Can you work these out from the model? Positions are in its coordinate system, mm. Face numbers are marked on the shaded views. Give positions to 0.01 mm unless a question says otherwise; leave off trailing zeros. Loops run counter-clockwise (first coordinate to the right, second up) from the corner with the lowest first, then second, coordinate; pieces in that order, holes last. Notation, with made-up numbers: (-16, -5) -> (0, -5) arc R10 cw to (0, 5) -> close; hole circle Ø10 at (62.25, 17). An arc over 180 degrees is marked (long way). One line per question, with ' | ' between items.
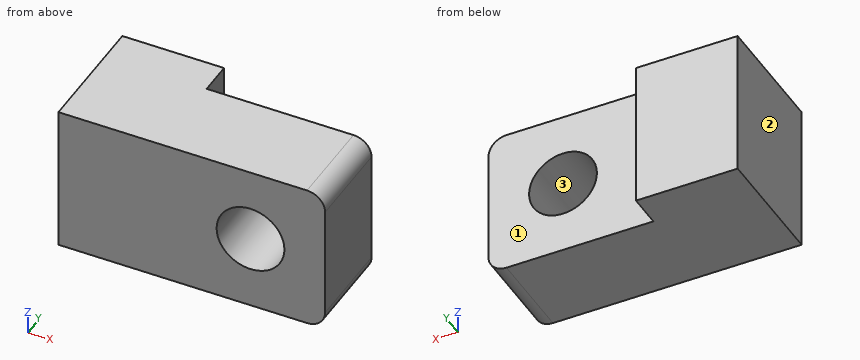
from build123d import *

# Parameters (mm, degrees)
SKETCH1_R           = 1.5
BOSS_EXTRUDE1_DEPTH = 4
SKETCH2_W           = 4.5
SKETCH2_H           = 6.6
BOSS_EXTRUDE2_DEPTH = 1.5


with BuildPart() as part:
    # Sketch1 → Boss-Extrude1 (new body)
    with BuildSketch(Plane(origin=(0, 0, 0), x_dir=(1, 0, 0), z_dir=(0, 1, 0))):
        with BuildLine():
            Line((11.8, -1), (11.8, -6))
            ThreePointArc((11.8, -6), (11.565685425, -6.565685425), (11, -6.8))
            Line((11, -6.8), (0, -6.8))
            Line((0, -6.8), (0, -0.2))
            Line((0, -0.2), (11, -0.2))
            ThreePointArc((11, -0.2), (11.565685425, -0.434314575), (11.8, -1))
        make_face()
        with Locations(Location((8.5, -3.5, 0), (0, 0, 270))):  # turned: the seam where the file's is
            Circle(SKETCH1_R, mode=Mode.SUBTRACT)
    extrude(amount=BOSS_EXTRUDE1_DEPTH)

    # Sketch2 → Boss-Extrude2 (add)
    with BuildSketch(Plane(origin=(0, 4, 0), x_dir=(1, 0, 0), z_dir=(0, 1, 0))):
        with Locations((2.25, -3.5)):
            Rectangle(SKETCH2_W, SKETCH2_H)
    extrude(amount=BOSS_EXTRUDE2_DEPTH)


solid = part.part
Q1. If we section it at C-C (z = 3.5): Write out the boundary of the cut face in (x, y), plus the area to 4 significant figures.
Entries:
outline: (0, 0) -> (7, 0) -> (7, 4) -> (4.5, 4) -> (4.5, 5.5) -> (0, 5.5) -> close; (10, 0) -> (11.8, 0) -> (11.8, 4) -> (10, 4) -> close | area: 41.95 mm²
Q2. If we section it at A-A (y = 1.1): Write out the boundary of the cut face in (x, z), plus the area to 3 significant figures.
Entries:
outline: (0, 0.2) -> (11, 0.2) arc R0.8 ccw to (11.8, 1) -> (11.8, 6) arc R0.8 ccw to (11, 6.8) -> (0, 6.8) -> close; hole circle Ø3 at (8.5, 3.5) | area: 70.5 mm²
Q3. If we section it at D-D (z = 5.5): Write out the boundary of the cut face in (x, y), plus the area to 4 significant figures.
Entries:
outline: (0, 0) -> (11.8, 0) -> (11.8, 4) -> (4.5, 4) -> (4.5, 5.5) -> (0, 5.5) -> close | area: 53.95 mm²
Q4. If we section it at B-B (x = 8.5): Write out the boundary of the cut face in (y, z), plus the area to 3 significant figures.
Entries:
outline: (0, 0.2) -> (4, 0.2) -> (4, 2) -> (0, 2) -> close; (0, 5) -> (4, 5) -> (4, 6.8) -> (0, 6.8) -> close | area: 14.4 mm²
Q5. If we mould it in two halves opening along X, with no side actions, what happens to the marked faces 1, 2 and 3? For each: pulls with the +X half, pulls with the -X half, needs draft (parallel to the pull), parting line crosses it, or undercut.
Entries:
face 1: needs draft | face 2: pulls with the -X half | face 3: undercut
Q6. If I drill on probe 1 along X at (y, z) = (0.95, 3.5); probe 2 along Y at (x, z) = (11, 3.5); probe 3 along X at (y, z) = (4.7, 5), over which ranges is the centre line in solid material (lowest first)? Write a range as from..to.
Entries:
probe 1: 0..7, 10..11.8 | probe 2: 0..4 | probe 3: 0..4.5
Q7. For pin 1 Ø1.2 at (y, z) = (5, 2.5) entering from +X, with a flat end and sliding along its axis, tell me the tip position at first contact or that it passes through.
Entries:
pin 1: x = 4.5
